from build123d import *

# Parameters (mm, degrees)
F1_DEPTH = 25.4
F2_W     = 19.05
F2_H     = 12.7
F3_DEPTH = 25.401
F4_T     = -2.54
F6_D     = 6.35
F6_DEPTH = 12.7


with BuildPart() as f1:
    # F0 (on Front) → F1 (new body)
    with BuildSketch(Plane.XZ):
        with BuildLine():
            ThreePointArc((0, 7.381471), (1.859872, 2.891343), (6.35, 1.031471))
            Line((6.35, 1.031471), (31.75, 1.031471))
            ThreePointArc((31.75, 1.031471), (36.240128, 2.891343), (38.1, 7.381471))
            Line((38.1, 7.381471), (38.1, 20.081471))
            ThreePointArc((38.1, 20.081471), (36.240128, 24.571599), (31.75, 26.431471))
            Line((31.75, 26.431471), (6.35, 26.431471))
            ThreePointArc((6.35, 26.431471), (1.859872, 24.571599), (0, 20.081471))
            Line((0, 20.081471), (0, 7.381471))
        make_face()
    extrude(amount=F1_DEPTH)

    # F2 (on face) → F3 (cut, through all)
    with BuildSketch(Plane.XZ.offset(25.4)):
        with Locations((19.05, 13.731471)):
            Rectangle(F2_W, F2_H)
    extrude(amount=-F3_DEPTH, mode=Mode.SUBTRACT)

    # F4
    f4_openings = [f1.faces().sort_by_distance(p)[0] for p in [
        (9.525, -12.7, 13.731471),
        (19.05, -12.7, 20.081471),
        (19.05, -12.7, 7.381471),
        (28.575, -12.7, 13.731471),
    ]]
    offset(amount=F4_T, openings=f4_openings)

    # F6
    with Locations(Plane.XY.offset(26.431471)):
        with Locations((12.636179, -6.286179), (25.463821, -19.113821)):
            Hole(F6_D / 2, depth=F6_DEPTH)


solid = f1.part
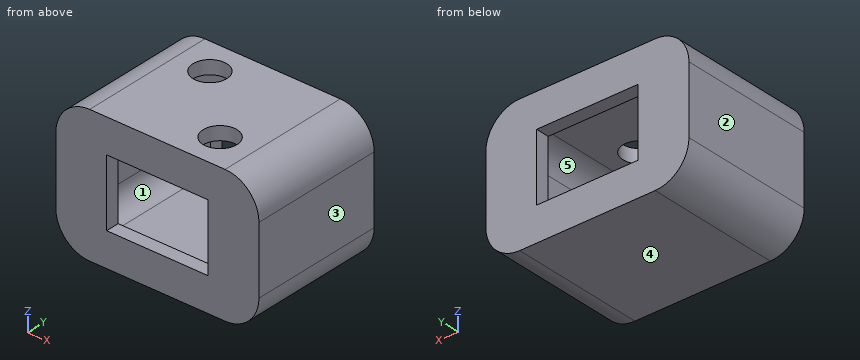
Check sheet for the modelled part. Datum: model origin and axes. Units: mm. Face numbers are marked on the shaded views. A direction names the side the tool comes from. Give positions to 0.01 mm unless a question says otherwise; leave off trailing zeros. Order: outer loops, then holes, each group sorted by start corner. A loop starts at its lowest first (then second) coordinate and runs counter-clockwise, first axis right, second up. Notation, with made-up numbers: M 27.25,22.25 L 33.25,22.25 A22 ccw 33.25,45.25 Z; hole C -2,-23.5 d8. An arc over 180 degrees is marked long. Answer as CSV lines item,"result". Start each with the question number.
Item 1: Cross-section at A-A on z = 8.5. Enter the section's corners in (x, y) (3 decimals), plus the area to 3 significant figures.
Item 2: Tool access check on the marked faces 1 and 2. Record the directions out of +Z, -Z, +X, -X, +Y, -Y that give a thin tool (end or side, any length) a straight path to the whole face; none if there is none.
Item 3: Thickness scan on line 1 (Z direction, x = 15.5, y = -4); line 2 (X direction, y = -18.5, z = 20.25); line 3 (Y direction, x = 17.5, z = 23.75). Record the ranges inside material, lowest first. Write a range as [from, to].
Item 4: Mould release check, pull along X, two halves, no side actions. Record for the marked faces 3, 4 and 5: +X half, -X half, draft (parallel to the pull), parting line (faces both ways), or undercut.
Item 5: Cross-section at B-B on x = 18.5. Enter the section's corners in (y, z).
Item 6: Cross-section at C-C on x = 30.5. Enter the section's corners in (y, z), plus the area to 3 significant figures.
Item 7: Cross-section at D-D on z = 5. Enter the section's corners in (x, y).
Established:
1,outline,"M 0,-25.4 L 9.525,-25.4 L 9.525,-22.86 L 2.54,-22.86 L 2.54,-2.54 L 9.525,-2.54 L 9.525,0 L 0,0 Z; M 28.575,-25.4 L 38.1,-25.4 L 38.1,0 L 28.575,0 L 28.575,-2.54 L 35.56,-2.54 L 35.56,-22.86 L 28.575,-22.86 Z"
1,area,"200 mm^2"
2,face 1,"none"
2,face 2,"+Z, -Z, -X, +Y, -Y"
3,line 1,"z = [1.03, 3.57], [23.89, 26.43]"
3,line 2,"x = [0, 2.54], [35.56, 38.1]"
3,line 3,"y = [-25.4, -22.86], [-2.54, 0]"
4,face 3,"+X half"
4,face 4,"draft"
4,face 5,"undercut"
5,outline,"M -25.4,1.03 L 0,1.03 L 0,7.38 L -2.54,7.38 L -2.54,3.57 L -22.86,3.57 L -22.86,7.38 L -25.4,7.38 Z; M -25.4,20.08 L -22.86,20.08 L -22.86,23.89 L -2.54,23.89 L -2.54,20.08 L 0,20.08 L 0,26.43 L -25.4,26.43 Z"
6,outline,"M -25.4,1.03 L 0,1.03 L 0,26.43 L -25.4,26.43 Z; hole M -22.86,3.57 L -2.54,3.57 L -2.54,23.89 L -22.86,23.89 Z"
6,area,"232 mm^2"
7,outline,"M 0.46,-25.4 L 37.64,-25.4 L 37.64,0 L 0.46,0 Z; hole M 3.38,-22.86 L 34.72,-22.86 L 34.72,-2.54 L 3.38,-2.54 Z"
